from build123d import *

# Parameters (mm, degrees)
F0_W     = 101.6
F0_H     = 25.4
F1_DEPTH = 101.6
F5_W     = 10
F5_H     = 10
F6_DEPTH = 25.401


with BuildPart() as f1:
    # F0 (on Front) → F1 (new body)
    with BuildSketch(Plane.XZ):
        with Locations((50.8, 12.7)):
            Rectangle(F0_W, F0_H)
    extrude(amount=-F1_DEPTH)

    # F2 (on face) → F4 section 0
    with BuildSketch(Plane.XZ):
        with BuildLine():
            Line((88.9, 25.4), (12.7, 25.4))
            ThreePointArc((12.7, 25.4), (50.8, 12.7), (88.9, 25.4))
        make_face()
    # F3 (on face) → F4 section 1
    with BuildSketch(Plane(origin=(0, 101.6, 0), x_dir=(-1, 0, 0), z_dir=(0, 1, 0))):
        with BuildLine():
            Line((-38.1, 25.4), (-63.5, 25.4))
            ThreePointArc((-63.5, 25.4), (-50.8, 15.24), (-38.1, 25.4))
        make_face()
    loft(mode=Mode.SUBTRACT)

    # F5 (on face) → F6 (cut, through all)
    with BuildSketch(Plane(origin=(0, 0, 0), x_dir=(1, 0, 0), z_dir=(0, 0, -1))):
        with Locations((50.8, -50.8)):
            Rectangle(F5_W, F5_H)
    extrude(amount=-F6_DEPTH, mode=Mode.SUBTRACT)


solid = f1.part
Read the model definition and answer for the solid it produces. Units are mm, in the model's axes. A direction names the side the tool comes from. Give positions to 0.01 mm unless a question says otherwise; leave off trailing zeros. Use CSV: the item, a comma, the result in double quotes. Start each with the question number.
(1) Given P1, Ø4, axis at x = 53.5, y = 45, coming from the +Z side, flat-ended and moving along its own axis, determine where the tip first touches the part or whether it passes through.
(2) Consider line 1 along Y through (x, z) = (55.5, 11.75); line 2 along X through (y, z) = (45, 18). Determine where each line is inside the solid, lowest interval first.
(3) Determine the mould class of faces 1 (the flat face through (55.8, 51, 7)), 2 (the flat face through (61, 50, 0)), 3 (the flat face through (101.6, 50, 13)), 4 (the flat face through (0, 50, 13)) for opening direction X: +X half, -X half, draft (parallel to the pull), parting line (faces both ways), or undercut.
(4) For faces 5 (the flat face through (87, 61, 25.4)), 6 (the flat face through (51, 45.8, 7)), determine the directions among +Z, -Z, +X, -X, +Y, -Y from which every point of the face is accessible in a straight line to the end or side of a thin tool.
Findings below:
1,P1,"z = 14.13"
2,line 1,"0 to 45.8, 55.8 to 101.6"
2,line 2,"0 to 33.72, 67.88 to 101.6"
3,face 1,"undercut"
3,face 2,"draft"
3,face 3,"+X half"
3,face 4,"-X half"
4,face 5,"+Z, +X, -X, +Y, -Y"
4,face 6,"+Z, -Z"
